```python
from build123d import *

# Parameters (mm, degrees)
F0_R     = 16
F1_DEPTH = 2
F2_R     = 1
F3_DEPTH = 12
F4_R     = 0.5


with BuildPart() as f1:
    # F0 (on Top) → F1 (new body)
    with BuildSketch(Plane.XY):
        Circle(F0_R)
        Polygon((10, 5.773503), (10, -5.773503), (0, -11.547005), (-10, -5.773503), (-10, 5.773503), (0, 11.547005), align=None, mode=Mode.SUBTRACT)
        Polygon((0, -11.547005), (10, -5.773503), (10, 5.773503), (0, 11.547005), (-10, 5.773503), (-10, -5.773503), align=None)
    extrude(amount=F1_DEPTH)

    # F2
    f2_edges = [f1.edges().sort_by_distance(p)[0] for p in [
        (-16, 0, 2),
    ]]
    fillet(f2_edges, radius=F2_R)

    # F0 (on Top) → F3 (join)
    with BuildSketch(Plane.XY):
        Polygon((0, -11.547005), (10, -5.773503), (10, 5.773503), (0, 11.547005), (-10, 5.773503), (-10, -5.773503), align=None)
    extrude(amount=F3_DEPTH)

    # F4
    f4_edges = [f1.edges().sort_by_distance(p)[0] for p in [
        (10, 0, 2),
        (5, -8.660254, 2),
        (10, -5.773503, 7),
        (10, 5.773503, 7),
        (5, 8.660254, 2),
        (0, 11.547005, 7),
        (-5, 8.660254, 2),
        (-10, 5.773503, 7),
        (-10, 0, 2),
        (-10, -5.773503, 7),
        (-5, -8.660254, 2),
        (0, -11.547005, 7),
    ]]
    fillet(f4_edges, radius=F4_R)


solid = f1.part
```
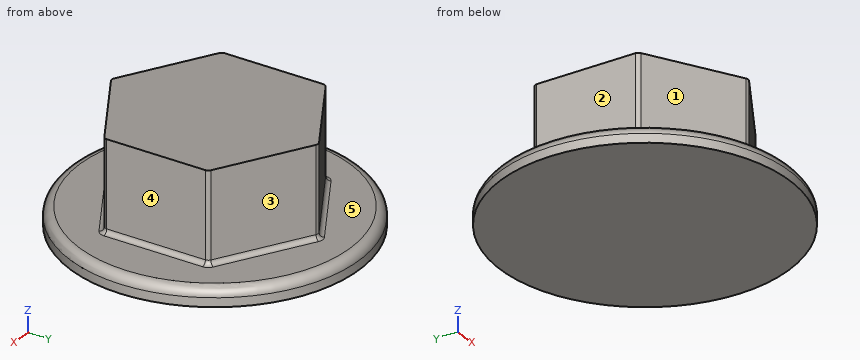
CAD build for the part. Positions are in the model's coordinates, mm. Face numbers are marked on the shaded views. A direction names the side the tool comes from. Coordinates: 2 decimals unless noted, no trailing zeros. Order: outer loops, then holes, each group sorted by start corner. A loop starts at its lowest first (then second) coordinate and runs counter-clockwise, first axis right, second up.
(1) Saw through at B-B, the plane z = 9.75. Write the cut outline in (x, y), and give its area (3 significant figures).
Solution:
outline: (-10, -5.48) arc R0.5 ccw to (-9.75, -5.92) - (-0.25, -11.4) arc R0.5 ccw to (0.25, -11.4) - (9.75, -5.92) arc R0.5 ccw to (10, -5.48) - (10, 5.48) arc R0.5 ccw to (9.75, 5.92) - (0.25, 11.4) arc R0.5 ccw to (-0.25, 11.4) - (-9.75, 5.92) arc R0.5 ccw to (-10, 5.48) - close
area: 346 mm2
(2) Pin check, flat tips, straight feed: pin 1 Ø3 at (y, z) = (0.5, 5) entering from +X; pin 2 Ø5 at (y, z) = (2.5, 5) entering from -X; pin 3 Ø4 at (y, z) = (12.5, 3) entering from +X. Stop position of each tip, or through.
Solution:
pin 1: stops at x = 10
pin 2: stops at x = -10
pin 3: stops at x = 11.27
(3) Which spindle directions (+Z, -Z, +X, -X, +Y, -Y) get a long thin tool onto all of the face, cutting with end or side? Do the marked faces 1, 2, 3, 4 and 5. Say none if no direction does.
Solution:
face 1: +Z, -X, -Y
face 2: +Z, -X, +Y, -Y
face 3: +Z, +X, +Y
face 4: +Z, +X, +Y, -Y
face 5: +Z
(4) Saw through at A-A, the plane y = 0. Write the cut outline in (x, z).
Solution:
outline: (-16, 0) - (16, 0) - (16, 1) arc R1 ccw to (15, 2) - (10.5, 2) arc R0.5 cw to (10, 2.5) - (10, 12) - (-10, 12) - (-10, 2.5) arc R0.5 cw to (-10.5, 2) - (-15, 2) arc R1 ccw to (-16, 1) - close
(5) Drill centre lines: L1, parallel to Z at x = 4.5, y = 10; L2, parallel to X at y = -0.5, z = 3.75; L3, parallel to Y at x = -7, z = 8.25. Where is each one in solid material? Low to high.
Solution:
L1: z = 0 to 2
L2: x = -10 to 10
L3: y = -7.51 to 7.51
